```python
from build123d import *

# Parameters (mm, degrees)
F0_W     = 1135.422638
F0_H     = 610.469668
F1_DEPTH = 10


with BuildPart() as f1:
    # F0 (on Top) → F1 (new body)
    with BuildSketch(Plane.XY):
        Polygon((614.296978, 355.234834), (-614.296978, 355.234834), (-974.371552, 355.234834), (-974.371552, 305.234834), (-614.296978, 305.234834), (-614.296978, -305.234834), (-974.371552, -305.234834), (-974.371552, -355.234834), (-614.296978, -355.234834), (614.296978, -355.234834), (927.263439, -355.234834), (927.263439, -305.234834), (614.296978, -305.234834), (614.296978, 305.234834), (927.263439, 305.234834), (927.263439, 355.234834), align=None)
        Rectangle(F0_W, F0_H, mode=Mode.SUBTRACT)
    extrude(amount=F1_DEPTH)


solid = f1.part
```
Verification items for the finished model (mm, model axes). Round coordinates to 2 decimals unless told otherwise and drop trailing zeros. Order: outer loops, then holes, each group sorted by start corner. A loop starts at its lowest first (then second) coordinate and runs counter-clockwise, first axis right, second up. Notation, with made-up numbers: (83.5, 12.25) -> (134.5, 12.25) arc R24 ccw to (134.5, 33.25) -> close; hole circle Ø1 at (-38, -32.75). An arc over 180 degrees is marked (long way). Put each result on its own line as item: value. Start each with the question number.
(1) Section check A-A (x = 677). Enter the section's corners in (y, z).
(2) Material ranges on line 1 along Y through (x, z) = (-374, 4.75); line 2 along X through (y, z) = (259, 4.5), recorded low to high.
(3) Depth check by flat-ended pin: pin 1 Ø5 at (y, z) = (-134, 6.5) entering from -X; pin 2 Ø5 at (y, z) = (-121.5, 7) entering from +X. Enter the tip coordinate at first touch or a pass-through.
(4) Section check C-C (z = 1.5). Enter the section's corners in (x, y), then the cut area to 3 significant figures.
(5) Draft check along Z on faces 1 (the face through (42, -314, 10)), 2 (the face through (42, -314, 0)). Enter one of: +Z half, -Z half, draft (parallel to the pull), parting line (faces both ways), or undercut.
(6) Section check B-B (y = -186). Enter the section's corners in (x, z), then the cut area to 3 significant figures.
Completed:
1. outline: (-355.23, 0) -> (-305.23, 0) -> (-305.23, 10) -> (-355.23, 10) -> close; (305.23, 0) -> (355.23, 0) -> (355.23, 10) -> (305.23, 10) -> close
2. line 1: y = -355.23 to -305.23, 305.23 to 355.23
2. line 2: x = -614.3 to -567.71, 567.71 to 614.3
3. pin 1: stops at x = -614.3
3. pin 2: stops at x = 614.3
4. outline: (-974.37, -355.23) -> (927.26, -355.23) -> (927.26, -305.23) -> (614.3, -305.23) -> (614.3, 305.23) -> (927.26, 305.23) -> (927.26, 355.23) -> (-974.37, 355.23) -> (-974.37, 305.23) -> (-614.3, 305.23) -> (-614.3, -305.23) -> (-974.37, -305.23) -> close; hole (-567.71, -305.23) -> (567.71, -305.23) -> (567.71, 305.23) -> (-567.71, 305.23) -> close
4. area: 247,000 mm2
5. face 1: +Z half
5. face 2: -Z half
6. outline: (-614.3, 0) -> (-567.71, 0) -> (-567.71, 10) -> (-614.3, 10) -> close; (567.71, 0) -> (614.3, 0) -> (614.3, 10) -> (567.71, 10) -> close
6. area: 932 mm2
